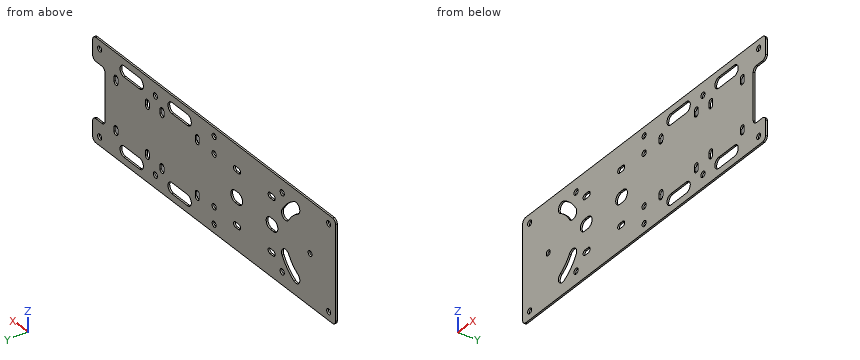
```python
from build123d import *

# Parameters (mm, degrees)
SKETCH1_W               = 392.54
SKETCH1_H               = 120
SKETCH1_R               = 3.2
BOSS_EXTRUDE1_DEPTH     = 2.03
CUT_EXTRUDE3_DEPTH      = 206.246275971
CUT_EXTRUDE3_DEPTH_BACK = 206.246275971
SKETCH3_R               = 3.15
CUT_EXTRUDE4_DEPTH      = 206.246275971
FILLET1_R               = 5
SKETCH4_R               = 3.35
CUT_EXTRUDE5_DEPTH      = 206.246275971


with BuildPart() as part:
    # Sketch1 → Boss-Extrude1 (new body)
    with BuildSketch(Plane(origin=(0, 0, 0), x_dir=(1, 0, 0), z_dir=(0, 1, 0))):
        Rectangle(SKETCH1_W, SKETCH1_H)
        with Locations(Location((0, -50, 0), (0, 0, 270))):
            Circle(SKETCH1_R, mode=Mode.SUBTRACT)
        with Locations(Location((185, -50, 0), (0, 0, 270))):
            Circle(SKETCH1_R, mode=Mode.SUBTRACT)
        with Locations(Location((185, 50, 0), (0, 0, 270))):
            Circle(SKETCH1_R, mode=Mode.SUBTRACT)
        with Locations(Location((0, 50, 0), (0, 0, 270))):
            Circle(SKETCH1_R, mode=Mode.SUBTRACT)
        with Locations(Location((-185, 50, 0), (0, 0, 270))):
            Circle(SKETCH1_R, mode=Mode.SUBTRACT)
        with Locations(Location((-185, -50, 0), (0, 0, 270))):
            Circle(SKETCH1_R, mode=Mode.SUBTRACT)
    extrude(amount=BOSS_EXTRUDE1_DEPTH)

    # Sketch2 → Cut-Extrude3 (cut, two sides: drawn at the far end of the back side and taken through both)
    with BuildSketch(Plane(origin=(0, 0, 0), x_dir=(1, 0, 0), z_dir=(0, 1, 0)).offset(-CUT_EXTRUDE3_DEPTH_BACK)):
        with BuildLine():
            Line((181.27, -32.5), (196.27, -32.5))
            Line((196.27, -32.5), (196.27, 32.5))
            Line((196.27, 32.5), (181.27, 32.5))
            ThreePointArc((181.27, 32.5), (177.734466094, 31.035533906), (176.27, 27.5))
            Line((176.27, 27.5), (176.27, -27.5))
            ThreePointArc((176.27, -27.5), (177.734466094, -31.035533906), (181.27, -32.5))
        make_face()
    extrude(amount=CUT_EXTRUDE3_DEPTH + CUT_EXTRUDE3_DEPTH_BACK, mode=Mode.SUBTRACT)

    # Sketch3 → Cut-Extrude4 (cut, through all)
    with BuildSketch(Plane(origin=(0, 0, 0), x_dir=(1, 0, 0), z_dir=(0, 1, 0))):
        with Locations(Location((-155, 0, 0), (0, 0, 270))):
            Circle(SKETCH3_R)
        with BuildLine():
            Line((-90.375, 34.83), (-95.535, 34.83))
            ThreePointArc((-95.535, 34.83), (-98.615, 31.75), (-95.535, 28.67))
            Line((-95.535, 28.67), (-90.375, 28.67))
            ThreePointArc((-90.375, 28.67), (-87.295, 31.75), (-90.375, 34.83))
        make_face()
        with BuildLine():
            Line((-39.625, 28.67), (-34.465, 28.67))
            ThreePointArc((-34.465, 28.67), (-31.385, 31.75), (-34.465, 34.83))
            Line((-34.465, 34.83), (-39.625, 34.83))
            ThreePointArc((-39.625, 34.83), (-42.705, 31.75), (-39.625, 28.67))
        make_face()
        with BuildLine():
            Line((-95.535, -34.83), (-90.375, -34.83))
            ThreePointArc((-90.375, -34.83), (-87.295, -31.75), (-90.375, -28.67))
            Line((-90.375, -28.67), (-95.535, -28.67))
            ThreePointArc((-95.535, -28.67), (-98.615, -31.75), (-95.535, -34.83))
        make_face()
        with BuildLine():
            Line((-39.625, -34.83), (-34.465, -34.83))
            ThreePointArc((-34.465, -34.83), (-31.385, -31.75), (-34.465, -28.67))
            Line((-34.465, -28.67), (-39.625, -28.67))
            ThreePointArc((-39.625, -28.67), (-42.705, -31.75), (-39.625, -34.83))
        make_face()
        with BuildLine():
            Line((24.14375, 29.25), (24.14375, 34.25))
            ThreePointArc((24.14375, 34.25), (27.14375, 37.25), (30.14375, 34.25))
            Line((30.14375, 34.25), (30.14375, 29.25))
            ThreePointArc((30.14375, 29.25), (27.14375, 26.25), (24.14375, 29.25))
        make_face()
        with BuildLine():
            Line((81.29375, 29.25), (81.29375, 34.25))
            ThreePointArc((81.29375, 34.25), (84.29375, 37.25), (87.29375, 34.25))
            Line((87.29375, 34.25), (87.29375, 29.25))
            ThreePointArc((87.29375, 29.25), (84.29375, 26.25), (81.29375, 29.25))
        make_face()
        with BuildLine():
            Line((24.14375, -34.25), (24.14375, -29.25))
            ThreePointArc((24.14375, -29.25), (27.14375, -26.25), (30.14375, -29.25))
            Line((30.14375, -29.25), (30.14375, -34.25))
            ThreePointArc((30.14375, -34.25), (27.14375, -37.25), (24.14375, -34.25))
        make_face()
        with BuildLine():
            Line((81.29375, -34.25), (81.29375, -29.25))
            ThreePointArc((81.29375, -29.25), (84.29375, -26.25), (87.29375, -29.25))
            Line((87.29375, -29.25), (87.29375, -34.25))
            ThreePointArc((87.29375, -34.25), (84.29375, -37.25), (81.29375, -34.25))
        make_face()
        with BuildLine():
            Line((104.7875, 26.075), (104.7875, 31.075))
            ThreePointArc((104.7875, 31.075), (107.7875, 34.075), (110.7875, 31.075))
            Line((110.7875, 31.075), (110.7875, 26.075))
            ThreePointArc((110.7875, 26.075), (107.7875, 23.075), (104.7875, 26.075))
        make_face()
        with BuildLine():
            Line((155.5875, 26.075), (155.5875, 31.075))
            ThreePointArc((155.5875, 31.075), (158.5875, 34.075), (161.5875, 31.075))
            Line((161.5875, 31.075), (161.5875, 26.075))
            ThreePointArc((161.5875, 26.075), (158.5875, 23.075), (155.5875, 26.075))
        make_face()
        with BuildLine():
            Line((104.7875, -31.075), (104.7875, -26.075))
            ThreePointArc((104.7875, -26.075), (107.7875, -23.075), (110.7875, -26.075))
            Line((110.7875, -26.075), (110.7875, -31.075))
            ThreePointArc((110.7875, -31.075), (107.7875, -34.075), (104.7875, -31.075))
        make_face()
        with BuildLine():
            Line((155.5875, -31.075), (155.5875, -26.075))
            ThreePointArc((155.5875, -26.075), (158.5875, -23.075), (161.5875, -26.075))
            Line((161.5875, -26.075), (161.5875, -31.075))
            ThreePointArc((161.5875, -31.075), (158.5875, -34.075), (155.5875, -31.075))
        make_face()
        with BuildLine():
            Line((120.6875, 51.9875), (145.6875, 51.9875))
            ThreePointArc((145.6875, 51.9875), (152.0375, 45.6375), (145.6875, 39.2875))
            Line((145.6875, 39.2875), (120.6875, 39.2875))
            ThreePointArc((120.6875, 39.2875), (114.3375, 45.6375), (120.6875, 51.9875))
        make_face()
        with BuildLine():
            Line((120.6875, -39.2875), (145.6875, -39.2875))
            ThreePointArc((145.6875, -39.2875), (152.0375, -45.6375), (145.6875, -51.9875))
            Line((145.6875, -51.9875), (120.6875, -51.9875))
            ThreePointArc((120.6875, -51.9875), (114.3375, -45.6375), (120.6875, -39.2875))
        make_face()
        with BuildLine():
            Line((43.21875, -39.2875), (68.21875, -39.2875))
            ThreePointArc((68.21875, -39.2875), (74.56875, -45.6375), (68.21875, -51.9875))
            Line((68.21875, -51.9875), (43.21875, -51.9875))
            ThreePointArc((43.21875, -51.9875), (36.86875, -45.6375), (43.21875, -39.2875))
        make_face()
        with BuildLine():
            Line((43.21875, 51.9875), (68.21875, 51.9875))
            ThreePointArc((68.21875, 51.9875), (74.56875, 45.6375), (68.21875, 39.2875))
            Line((68.21875, 39.2875), (43.21875, 39.2875))
            ThreePointArc((43.21875, 39.2875), (36.86875, 45.6375), (43.21875, 51.9875))
        make_face()
        with BuildLine():
            Line((-96.105, 6.85), (-90.945, 6.85))
            ThreePointArc((-90.945, 6.85), (-84.095, 0), (-90.945, -6.85))
            Line((-90.945, -6.85), (-96.105, -6.85))
            ThreePointArc((-96.105, -6.85), (-102.955, 0), (-96.105, 6.85))
        make_face()
        with BuildLine():
            Line((-33.895, -6.85), (-39.055, -6.85))
            ThreePointArc((-39.055, -6.85), (-45.905, 0), (-39.055, 6.85))
            Line((-39.055, 6.85), (-33.895, 6.85))
            ThreePointArc((-33.895, 6.85), (-27.045, 0), (-33.895, -6.85))
        make_face()
        with BuildLine():
            ThreePointArc((-135.25, -34.208003449), (-127.069282143, -27.930717857), (-120.791996551, -19.75))
            ThreePointArc((-120.791996551, -19.75), (-112.117735236, -17.425738686), (-109.793473922, -26.1))
            ThreePointArc((-109.793473922, -26.1), (-118.089026022, -36.910973978), (-128.9, -45.206526078))
            ThreePointArc((-128.9, -45.206526078), (-137.574261314, -42.882264764), (-135.25, -34.208003449))
        make_face()
        with BuildLine():
            ThreePointArc((-128.9, 45.206526078), (-137.574261314, 42.882264764), (-135.25, 34.208003449))
            ThreePointArc((-135.25, 34.208003449), (-127.069282143, 27.930717857), (-120.791996551, 19.75))
            ThreePointArc((-120.791996551, 19.75), (-112.117735236, 17.425738686), (-109.793473922, 26.1))
            ThreePointArc((-109.793473922, 26.1), (-118.089026022, 36.910973978), (-128.9, 45.206526078))
        make_face()
    extrude(amount=CUT_EXTRUDE4_DEPTH, mode=Mode.SUBTRACT)

    # Fillet1
    fillet1_edges = [part.edges().sort_by_distance(p)[0] for p in [
        (196.27, 1.015, -32.5),
        (196.27, 1.015, 32.5),
        (196.27, 1.015, 60),
        (-196.27, 1.015, 60),
        (-196.27, 1.015, -60),
        (196.27, 1.015, -60),
    ]]
    fillet(fillet1_edges, radius=FILLET1_R)

    # Sketch4 → Cut-Extrude5 (cut, through all)
    with BuildSketch(Plane(origin=(0, 2.03, 0), x_dir=(1, 0, 0), z_dir=(0, 1, 0))):
        with Locations(Location((-110, 45, 0), (0, 0, 270))):
            Circle(SKETCH4_R)
        with Locations(Location((0, 30, 0), (0, 0, 270))):
            Circle(SKETCH4_R)
        with Locations(Location((95, 45, 0), (0, 0, 270))):
            Circle(SKETCH4_R)
        with Locations(Location((95, -45, 0), (0, 0, 90))):
            Circle(SKETCH4_R)
        with Locations(Location((0, -30, 0), (0, 0, 90))):
            Circle(SKETCH4_R)
        with Locations(Location((-110, -45, 0), (0, 0, 90))):
            Circle(SKETCH4_R)
    extrude(amount=-CUT_EXTRUDE5_DEPTH, mode=Mode.SUBTRACT)


solid = part.part
```
Model file for the job. Use its own axes, mm. Give positions to 0.01 mm unless a question says otherwise; leave off trailing zeros. Use CSV: the item, a comma, the result in double quotes. Start each with the question number.
1) Wall check: line 1 (Z direction, x = -0.5, y = 1); line 2 (X direction, y = 0.4, z = 50); line 3 (Z direction, x = 181, y = 1). Give the ranges that are in metal, low to high.
2) Slice it at A-A on y = 1.05. Give the number of separate pieces and of enclosed holes in the cut face, plus the area to 3 significant figures.
3) Flat gauge pins, fed straight in: pin 1 Ø1 at (y, z) = (1, 8.5) entering from +X; pin 2 Ø7 at (x, z) = (-155, 0) entering from -Y; pin 3 Ø5 at (x, z) = (185, -50) entering from +Y; pin 4 Ø1 at (y, z) = (1, -31.5) entering from +X. Where does each tip first touch, or does it go through?
Computed values:
1,line 1,"z = -60 to -53.16, -46.84 to -33.31, -26.69 to 26.69, 33.31 to 46.84, 53.16 to 60"
1,line 2,"x = -196.27 to -188.2, -181.8 to -3.2, 3.2 to 38.6, 72.83 to 116.07, 150.3 to 181.8, 188.2 to 196.27"
1,line 3,"z = -60 to -32.49, 32.49 to 60"
2,separate pieces,"1"
2,enclosed holes,"33"
2,area,"41,600 mm^2"
3,pin 1,"stops at x = 176.27"
3,pin 2,"stops at y = 0"
3,pin 3,"passes through"
3,pin 4,"stops at x = 179.09"
